For this review, take the finished solid that the model builds, in its own axes (mm). A direction names the side the tool comes from. Round coordinates to 2 decimals unless told otherwise and drop trailing zeros. Loops run counter-clockwise (first coordinate to the right, second up) from the corner with the lowest first, then second, coordinate; pieces in that order, holes last. Notation, with made-up numbers: (-24, -17) -> (-5, -17) arc R31 ccw to (-5, 8) -> close; hole circle Ø6 at (72, 89.5). An arc over 180 degrees is marked (long way). Use one line per item in the form item = value. Start each with the question number.
from build123d import *

# Parameters (mm, degrees)
CROQUIS1_W              = 24.3
CROQUIS1_H              = 24.3
CROQUIS1_W_2            = 20.3
CROQUIS1_H_2            = 20.3
SALIENTE_EXTRUIR1_DEPTH = 35
CROQUIS2_R              = 2.15
SALIENTE_EXTRUIR2_DEPTH = 3
CROQUIS3_R              = 2.15
SALIENTE_EXTRUIR3_DEPTH = 3
SALIENTE_EXTRUIR4_DEPTH = 1
CROQUIS5_R              = 2.1
CORTAR_EXTRUIR1_DEPTH   = 28.65


with BuildPart() as part:
    # Croquis1 → Saliente-Extruir1 (new body, symmetric)
    with BuildSketch(Plane.XY):
        Rectangle(CROQUIS1_W, CROQUIS1_H)
        Rectangle(CROQUIS1_W_2, CROQUIS1_H_2, mode=Mode.SUBTRACT)
    extrude(amount=SALIENTE_EXTRUIR1_DEPTH, both=True)

    # Croquis2 → Saliente-Extruir2 (add)
    with BuildSketch(Plane.XY.offset(35)):
        Polygon((15.5, -12.15), (15.5, 27), (15.5, 31.15), (-15.5, 31.15), (-15.5, -12.15), (-12.15, -12.15), (-12.15, 12.15), (12.15, 12.15), (12.15, -12.15), align=None)
        with Locations((-11.35, 27)):
            Circle(CROQUIS2_R, mode=Mode.SUBTRACT)
        with Locations((11.35, 27)):
            Circle(CROQUIS2_R, mode=Mode.SUBTRACT)
    extrude(amount=-SALIENTE_EXTRUIR2_DEPTH)

    # Croquis3 → Saliente-Extruir3 (add)
    with BuildSketch(Plane(origin=(0, 0, -35), x_dir=(-1, 0, 0), z_dir=(0, 0, -1))):
        Polygon((12.15, -12.15), (15.5, -12.15), (15.5, 57.5), (6.9, 57.5), (-15.5, 31.15), (-15.5, -12.15), (-12.15, -12.15), (-12.15, 12.15), (12.15, 12.15), align=None)
        with Locations((11.05, 53.35)):
            Circle(CROQUIS3_R, mode=Mode.SUBTRACT)
        with Locations((11.05, 46.35)):
            Circle(CROQUIS3_R, mode=Mode.SUBTRACT)
    extrude(amount=-SALIENTE_EXTRUIR3_DEPTH)

    # Croquis4 → Saliente-Extruir4 (add, symmetric)
    with BuildSketch(Plane(origin=(0, 0, 0), x_dir=(0, 0, -1), z_dir=(1, 0, 0))):
        Polygon((-32, 12.15), (32, 12.15), (32, 47.15), (-32, 31.15), align=None)
    extrude(amount=SALIENTE_EXTRUIR4_DEPTH, both=True)

    # Croquis5 → Cortar-Extruir1 (cut, through all)
    with BuildSketch(Plane(origin=(12.15, 0, 0), x_dir=(0, 0, -1), z_dir=(1, 0, 0))):
        with Locations((-16, 0)):
            Circle(CROQUIS5_R)
        with Locations((16, 0)):
            Circle(CROQUIS5_R)
    extrude(amount=-CORTAR_EXTRUIR1_DEPTH, mode=Mode.SUBTRACT)


solid = part.part
Item 1: For P1, Ø5, axis at y = 11, z = -1, coming from the +X side; P2, Ø9, axis at x = 8, z = 8.5, coming from the +Y side; P3, Ø2, axis at x = -9.5, y = 46.5, coming from the +Z side; P4, Ø10, axis at y = 50.5, z = -6, coming from the +X side, all flat-tipped, find the tip position at first contact; note any pin that passes through.
Item 2: Take a section at D-D on y = 27. Give the boundary of the cut face in (x, z), plus the area to 3 significant figures.
Item 3: Draft analysis for pull direction Y (two halves, no side actions). For faces 1 (the flat face through (-15.5, 22, -34)), 2 (the cylindrical face through (-11.14, 0.09, -13.9)), 3 (the flat face through (-7, 12.15, 0)), state which applies: +Y half, -Y half, draft (parallel to the pull), parting line (faces both ways), or undercut.
Item 4: Machinability: for faces 4 (the flat face through (1, 26, 0)), 5 (the flat face through (0, 10.15, 0)), 6 (the flat face through (0, 31.15, 34)), which of the approach directions +Z, -Z, +X, -X, +Y, -Y give a long, thin tool a straight path to every point of the face, cutting with its end or side? Answer none if there is none.
Item 5: Take a section at C-C on x = 11. Give the boundary of the cut face in (y, z), plus the area to 3 significant figures.
Item 6: Wall thickness on line 1 (Y direction, x = -11, z = -33); line 2 (Y direction, x = -7, z = -10); line 3 (Z direction, x = -12, y = 18): over which ranges is each line inside the solid? List them lowest first.
Item 7: Take a section at B-B on y = -4.5. Give the boundary of the cut face in (x, z), plus the area to 3 significant figures.
Item 8: Take a section at A-A on z = -16. Give the boundary of the cut face in (x, y).
Results:
q1.P1 = 12.15
q1.P2 = 12.15
q1.P3 = -32
q1.P4 = through
q2.outline = (-15.5, -35) -> (15.5, -35) -> (15.5, -32) -> (1, -32) -> (1, 32) -> (9.2, 32) -> (9.2, 35) -> (-9.2, 35) -> (-9.2, 32) -> (-1, 32) -> (-1, -32) -> (-15.5, -32) -> close; (-15.5, 32) -> (-13.5, 32) -> (-13.5, 35) -> (-15.5, 35) -> close; (13.5, 32) -> (15.5, 32) -> (15.5, 35) -> (13.5, 35) -> close
q2.area = 288 mm2
q3.face_1 = draft
q3.face_2 = undercut
q3.face_3 = +Y half
q4.face_4 = +X, +Y
q4.face_5 = +Z, -Z
q4.face_6 = +Z, +X, -X, +Y
q5.outline = (-12.15, -35) -> (36.44, -35) -> (36.44, -32) -> (12.15, -32) -> (12.15, 32) -> (24.88, 32) -> (24.88, 35) -> (-12.15, 35) -> close; (29.12, 32) -> (31.15, 32) -> (31.15, 35) -> (29.12, 35) -> close; hole circle Ø4.2 at (0, -16); hole circle Ø4.2 at (0, 16)
q5.area = 1,790 mm2
q6.line_1 = -12.15 to 44.2, 48.5 to 51.2, 55.5 to 57.5
q6.line_2 = -12.15 to -10.15, 10.15 to 12.15
q6.line_3 = -35 to -32, 32 to 35
q7.outline = (-15.5, -35) -> (-10.15, -35) -> (-10.15, 35) -> (-15.5, 35) -> (-15.5, 32) -> (-12.15, 32) -> (-12.15, -32) -> (-15.5, -32) -> close; (10.15, -35) -> (15.5, -35) -> (15.5, -32) -> (12.15, -32) -> (12.15, 32) -> (15.5, 32) -> (15.5, 35) -> (10.15, 35) -> close
q7.area = 320 mm2
q8.outline = (-12.15, -12.15) -> (12.15, -12.15) -> (12.15, -2.1) -> (10.15, -2.1) -> (10.15, -10.15) -> (-10.15, -10.15) -> (-10.15, -2.1) -> (-12.15, -2.1) -> close; (-12.15, 2.1) -> (-10.15, 2.1) -> (-10.15, 10.15) -> (10.15, 10.15) -> (10.15, 2.1) -> (12.15, 2.1) -> (12.15, 12.15) -> (1, 12.15) -> (1, 43.15) -> (-1, 43.15) -> (-1, 12.15) -> (-12.15, 12.15) -> close
